Source: CAD feature listing. Evaluate the final solid. Frame: model axes, mm. Give positions to 0.01 mm unless a question says otherwise; leave off trailing zeros. Write each loop counter-clockwise with the first axis right and the second up, starting at its lowest first coordinate (ties: lowest second). Pieces come first, ordered by that corner, then holes. Notation, with made-up numbers: (-3.75, 10) -> (17.25, 10) arc R23 ccw to (17.25, 41) -> close; hole circle Ø5 at (-11.5, 19.5). An arc over 180 degrees is marked (long way). Write item = value, one per line.
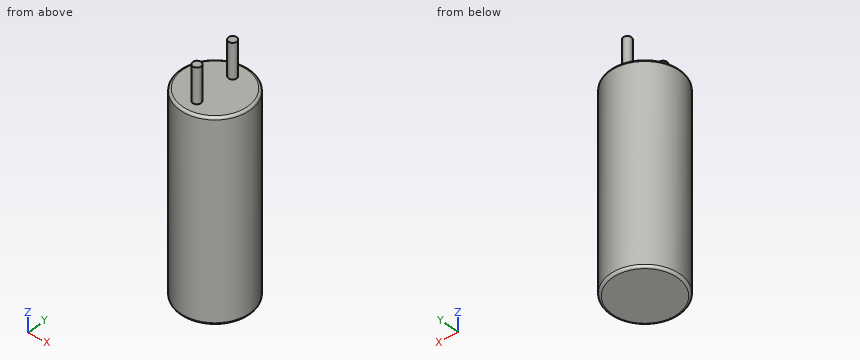
Autodesk Inventor part; units mm, degrees
ref_plane "YZ Plane" through (0, 0, 0) normal (1, 0, 0) x (0, 1, 0)
ref_plane "XZ Plane" through (0, 0, 0) normal (0, 1, 0) x (-1, 0, 0)
ref_plane "XY Plane" through (0, 0, 0) normal (0, 0, 1) x (1, 0, 0)
sketch "Эскиз1" plane through (0, 0, 0) normal (0, 0, 1) x (1, 0, 0)
  circle A0 centre (0, 0) radius 3
  circle A1 centre (0, 1.6837) radius 0.3522
  circle A2 centre (0, -1.7307) radius 0.3546
  dimension "d0" = 6
extrude "Выдавливание1" add sketch "Эскиз1" against normal blind 17 contours A0 | A1 | A2
extrude "Выдавливание2" add sketch "Эскиз1" along normal blind 3 contours A1 | A2
fillet "Сопряжение1" radius 0.2 2 edges at (-3, 0, 0) (-3, 0, -17)
properties part number "термодатчик"
(1) Section query C-C (z = 0.75). Return loops of the section in (x, y).
Values follow:
outline = circle Ø0.71 at (0, -1.73); circle Ø0.7 at (0, 1.68)
(2) Section query B-B (x = 0). Return loops of the section in (y, z).
Values follow:
outline = (-3, -16.8) arc R0.2 ccw to (-2.8, -17) -> (2.8, -17) arc R0.2 ccw to (3, -16.8) -> (3, -0.2) arc R0.2 ccw to (2.8, 0) -> (2.04, 0) -> (2.04, 3) -> (1.33, 3) -> (1.33, 0) -> (-1.38, 0) -> (-1.38, 3) -> (-2.09, 3) -> (-2.09, 0) -> (-2.8, 0) arc R0.2 ccw to (-3, -0.2) -> close
(3) First-contact query: pin 1 (1 mm diameter, centred on x = -1, y = 1.5, fed in from +Z); pin 2 (1 mm diameter, centred on x = -2, z = -10.5, fed in from -Y); pin 3 (1.5 mm diameter, centred on y = 2.5, z = -8.5, fed in from +X). Flat tips, straight axial feed; report the tip coordinate or a pass-through.
Values follow:
pin_1 = 0
pin_2 = -2.6
pin_3 = 2.44
(4) Section query A-A (y = 0). Return loops of the section in (x, z), plus the area to 3 significant figures.
Values follow:
outline = (-3, -16.8) arc R0.2 ccw to (-2.8, -17) -> (2.8, -17) arc R0.2 ccw to (3, -16.8) -> (3, -0.2) arc R0.2 ccw to (2.8, 0) -> (-2.8, 0) arc R0.2 ccw to (-3, -0.2) -> close
area = 102 mm2
(5) Material intervals for line 1 (Z direction, x = -1.25, y = 1.25); line 2 (Y direction, x = -1.5, z = -11); line 3 (X direction, y = -2, z = -2), sorted ascending.
Values follow:
line_1 = -17 to 0
line_2 = -2.6 to 2.6
line_3 = -2.24 to 2.24
(6) Section query D-D (z = -6). Return loops of the section in (x, y).
Values follow:
outline = circle Ø6 at (0, 0)
